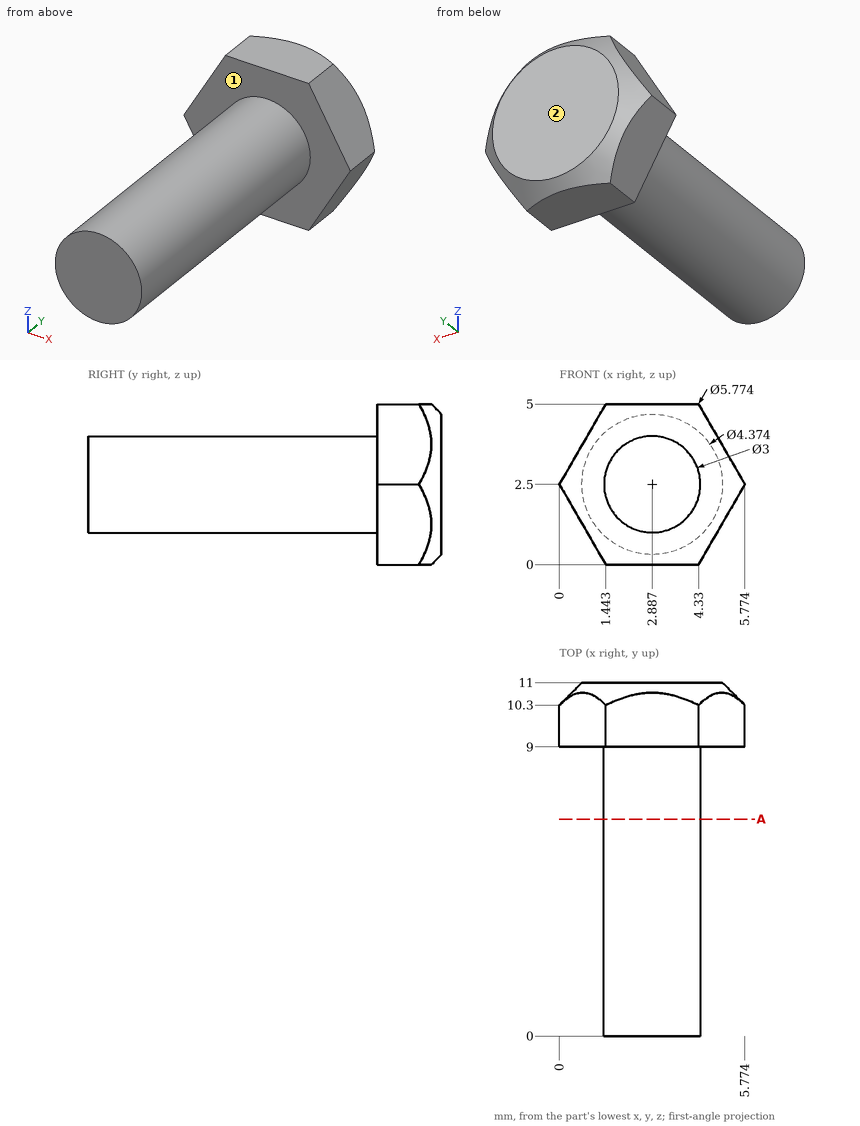
The figure shows three views and two pictorial views of one solid part (mm, origin at its lowest corner). Answer the questions. A direction names the side the tool comes from. Give positions to 0.01 mm unless a question says otherwise; leave off trailing zeros. Order: outer loops, then holes, each group sorted by start corner. A loop starts at its lowest first (then second) coordinate and runs counter-clockwise, first axis right, second up. Notation, with made-up numbers: M 65.25,24.5 L 79.25,24.5 A23 ccw 79.25,46.5 Z; hole C 55,-27 d6. An arc over 180 degrees is marked long. Return JSON: item names as keys, results as strings.
Q1. Each of these flat-tipped pins is pushed along its axis until it touches: pin 1 (3 mm diameter, centred on y = 8, z = 3.5, fed in from +X); pin 2 (3 mm diameter, centred on y = 3, z = 3.5, fed in from +X); pin 3 (1.5 mm diameter, centred on y = 5, z = 1, fed in from -X). Where does it stop, or does it pass through?
Answer below:
{"pin 1": "stops at x = 5.77", "pin 2": "stops at x = 4.39", "pin 3": "stops at x = 1.59"}
Q2. Find the intervals of material crossed by line 1 along X through (y, z) = (2.25, 2.9); line 2 along Y through (x, z) = (2.15, 4.35); line 3 along Z through (x, y) = (1.95, 7.25), in increasing order. Write a range as [from, to].
Answer below:
{"line 1": "x = [1.44, 4.33]", "line 2": "y = [9, 11]", "line 3": "z = [1.33, 3.67]"}
Q3. Which of the six approach directions +Z, -Z, +X, -X, +Y, -Y give full straight-line access (tool end or side, diameter ignored) to the marked faces 1 and 2?
Answer below:
{"face 1": "-Y", "face 2": "+Z, -Z, +X, -X, +Y"}
Q4. Find section A-A, the plane y = 6.75. Write down the section's boundary in (x, z).
Answer below:
{"outline": "C 2.89,2.5 d3"}
